Build history of the part. All positions in model axes, mm. Face numbers are marked on the shaded views. Round coordinates to 2 decimals unless told otherwise and drop trailing zeros. Loops run counter-clockwise (first coordinate to the right, second up) from the corner with the lowest first, then second, coordinate; pieces in that order, holes last. Notation, with made-up numbers: (15, 11) - (39, 11) arc R25 cw to (39, 39) - close; hole circle Ø6 at (75, 79.25). An arc over 180 degrees is marked (long way). Use one line per item in the form item = value. Start each with the question number.
Q1. Drill centre lines: line 1 (Y direction, x = 0, z = 2.5); line 2 (Y direction, x = 0, z = 2.75); line 3 (Z direction, x = -7.5, y = -7). Where is each one in solid material? Low to high.
Q2. Pin check, flat tips, straight feed: pin 1 (3 mm diameter, centred on y = 11.5, z = 7.5, fed in from -X); pin 2 (3 mm diameter, centred on y = -1.5, z = 7, fed in from +X); pin 3 (12 mm diameter, centred on x = 3.5, y = -7.5, fed in from -Z); pin 4 (2 mm diameter, centred on x = 4, z = 3, fed in from +Y). Stop position of each tip, or through.
Q3. Saw through at D-D (z = 1). Give the cut face in (x, y), then the cut area to 3 significant figures.
Q4. Mould opens along Y. For the marked faces 1 and 2 say: released by +Y, released by -Y, zero draft, split by the parting line, or undercut.
Q5. Saw through at C-C (z = 5.75). Give the cut face in (x, y), then the cut area to 3 significant figures.
```python
from build123d import *

# Parameters (mm, degrees)
SKETCH1_R           = 15
BOSS_EXTRUDE1_DEPTH = 10
FILLET1_R           = 5
FILLET2_R           = 5
SKETCH2_R           = 1.5
CUT_EXTRUDE1_DEPTH  = 24.452078799


with BuildPart() as part:
    # Sketch1 → Boss-Extrude1 (new body)
    with BuildSketch(Plane.XY):
        Circle(SKETCH1_R)
    extrude(amount=BOSS_EXTRUDE1_DEPTH)

    # Fillet1
    fillet1_edges = [part.edges().sort_by_distance(p)[0] for p in [
        (-15, 0, 10),
    ]]
    fillet(fillet1_edges, radius=FILLET1_R)

    # Fillet2
    fillet2_edges = [part.edges().sort_by_distance(p)[0] for p in [
        (-15, 0, 0),
    ]]
    fillet(fillet2_edges, radius=FILLET2_R - 0.0001)  # a hair under: the kernel refuses the full size

    # Sketch2 → Cut-Extrude1 (cut, through all)
    with BuildSketch(Plane.XY.offset(10)):
        Circle(SKETCH2_R)
    extrude(amount=-CUT_EXTRUDE1_DEPTH, mode=Mode.SUBTRACT)


solid = part.part
```
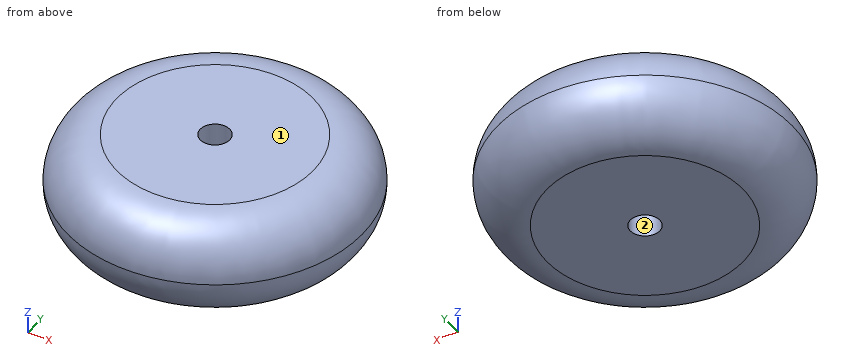
Report:
q1.line_1 = -14.33 to -1.5, 1.5 to 14.33
q1.line_2 = -14.47 to -1.5, 1.5 to 14.47
q1.line_3 = 0.01 to 9.99
q2.pin_1 = -10.56
q2.pin_2 = 14.93
q2.pin_3 = 0
q2.pin_4 = 14.46
q3.outline = circle Ø26 at (0, 0); hole circle Ø3 at (0, 0)
q3.area = 524 mm²
q4.face_1 = zero draft
q4.face_2 = undercut
q5.outline = circle Ø29.89 at (0, 0); hole circle Ø3 at (0, 0)
q5.area = 694 mm²
